Geometry: final body of the model. Coordinates: model frame, mm. A direction names the side the tool comes from. Give positions to 0.01 mm unless a question says otherwise; leave off trailing zeros. Write each loop counter-clockwise with the first axis right and the second up, starting at its lowest first coordinate (ties: lowest second). Pieces come first, ordered by that corner, then holes. Notation, with made-up numbers: (66, 81.25) -> (104, 81.25) arc R13 ccw to (104, 101.25) -> close; hole circle Ø4 at (47, -31.5). An arc over 180 degrees is marked (long way). Answer in a Markdown table with one row per item. Add a question column.
Item 1: Material intervals for probe 1 along X at (y, z) = (14, -23); probe 2 along Y at (x, z) = (-9.75, 12); probe 3 along Z at (x, y) = (-0.75, 15), sorted ascending. Write a range as from..to.
Item 2: Section query B-B on y = 20.25. Output: boundary loops of the cut face in (x, z), plus the area to 3 significant figures.
Item 3: Section query C-C on x = -1.75. Output: boundary loops of the cut face in (y, z).
Item 4: First-contact query: P1, Ø8, axis at x = -9, y = 6.5, coming from the -Z side; P2, Ø6, axis at x = -8, z = -9, coming from the +Y side; P3, Ø4, axis at y = 15, z = -12, coming from the +X side; P4, Ø3, axis at x = 11, y = 16.5, coming from the -Z side. Flat tips, straight axial feed; report the tip coordinate or a pass-through.
Item 5: Section query D-D on y = 15. Output: boundary loops of the cut face in (x, z).
Item 6: Draft query along Y for faces 1 (the flat face through (-0.133, 25.244, 25.986)), 2 (the flat face through (7.5, 16, 0)), 3 (the cylindrical face through (-11.2, 12.87, -14.32)), 4 (the flat face through (0, 0, 0)). Return one class per face: +Y half, -Y half, draft (parallel to the pull), parting line (faces both ways), or undercut.
Item 7: Section query A-A on z = 12.5. Output: boundary loops of the cut face in (x, y), plus the area to 3 significant figures.
Item 8: Access query for faces 5 (the flat face through (0, 21, -25)), 6 (the flat face through (-15, 16, 1)). Directions: +Z, -Z, +X, -X, +Y, -Y. A direction counts if a zero-diameter tool reaches every point of the face in a straight line with its end or side. Return the directions, or none.
```python
from build123d import *

# Parameters (mm, degrees)
SKETCH1_W           = 30
SKETCH1_H           = 80
BOSS_EXTRUDE1_DEPTH = 27
SKETCH5_W           = 30
SKETCH5_H           = 10
BOSS_EXTRUDE2_DEPTH = 6
SKETCH2_R           = 3.15
CUT_EXTRUDE1_DEPTH  = 40
FILLET5_R           = 40
FILLET6_R           = 40
FILLET7_R           = 2
FILLET8_R           = 2
SKETCH6_W           = 10
SKETCH6_H           = 6
CUT_EXTRUDE2_DEPTH  = 60.301649892
SKETCH7_W           = 15
SKETCH7_H           = 50
CUT_EXTRUDE3_DEPTH  = 19
FILLET9_R           = 10
CHAMFER1_SIZE       = 2
CHAMFER1_SIZE2      = 3.464101615


with BuildPart() as part:
    # Sketch1 → Boss-Extrude1 (new body)
    with BuildSketch(Plane(origin=(0, 0, 0), x_dir=(1, 0, 0), z_dir=(0, 1, 0))):
        Rectangle(SKETCH1_W, SKETCH1_H)
    extrude(amount=BOSS_EXTRUDE1_DEPTH)

    # Sketch5 → Boss-Extrude2 (add)
    with BuildSketch(Plane(origin=(0, 27, 0), x_dir=(1, 0, 0), z_dir=(0, 1, 0))):
        Rectangle(SKETCH5_W, SKETCH5_H)
    extrude(amount=BOSS_EXTRUDE2_DEPTH)

    # Sketch2 → Cut-Extrude1 (cut)
    with BuildSketch(Plane(origin=(15, 0, 0), x_dir=(0, 0, -1), z_dir=(1, 0, 0))):
        with Locations((-12, 15)):
            Circle(SKETCH2_R)
        with Locations(Location((12, 15, 0), (0, 0, 180))):
            Circle(SKETCH2_R)
    extrude(amount=-CUT_EXTRUDE1_DEPTH, mode=Mode.SUBTRACT)

    # Fillet5
    # the kernel refuses this fillet: 40 mm, written as the material it takes off along each edge
    with BuildSketch(Plane(origin=(109.571401597, 0, -40), x_dir=(0, 0, 1), z_dir=(-1, 0, 0))) as fillet5_piece_1:
        with BuildLine():
            CenterArc((37.828560639, 40), FILLET5_R, 198.965574989, 71.034425011)
            Line((0, 27), (-0.756571213, 26.74))
            ThreePointArc((-0.756571213, 26.74), (-0.8, 13.5), (-0.8, 0))
            Line((-0.8, 0), (0, -0.8))
            Line((0, -0.8), (37.828560639, -0.8))
            Line((37.828560639, -0.8), (37.828560639, 0))
        make_face()
    extrude(amount=219.142803194, mode=Mode.SUBTRACT)

    # Fillet6
    # the kernel refuses this fillet: 40 mm, written as the material it takes off along each edge
    with BuildSketch(Plane(origin=(-109.571401597, 0, 40), x_dir=(0, 1, 0), z_dir=(1, 0, 0))) as fillet6_piece_1:
        with BuildLine():
            CenterArc((40, -37.828560639), FILLET6_R, 108.965574989, 71.034425011)
            Line((0, -37.828560639), (-0.8, -37.828560639))
            Line((-0.8, -37.828560639), (-0.8, 0))
            Line((-0.8, 0), (0, 0.8))
            ThreePointArc((0, 0.8), (13.5, 0.8), (26.74, 0.756571213))
            Line((26.74, 0.756571213), (27, 0))
        make_face()
    extrude(amount=219.142803194, mode=Mode.SUBTRACT)

    # Fillet7
    fillet7_edges = [part.edges().sort_by_distance(p)[0] for p in [
        (0, 27, -40),
    ]]
    fillet(fillet7_edges, radius=FILLET7_R)

    # Fillet8
    fillet8_edges = [part.edges().sort_by_distance(p)[0] for p in [
        (0, 27, 40),
    ]]
    fillet(fillet8_edges, radius=FILLET8_R)

    # Sketch6 → Cut-Extrude2 (cut, through all)
    with BuildSketch(Plane(origin=(15, 0, 0), x_dir=(0, 0, -1), z_dir=(1, 0, 0))):
        with Locations((0, 30)):
            Rectangle(SKETCH6_W, SKETCH6_H)
    extrude(amount=-CUT_EXTRUDE2_DEPTH, mode=Mode.SUBTRACT)

    # Sketch7 → Cut-Extrude3 (cut)
    with BuildSketch(Plane(origin=(0, 27, 0), x_dir=(1, 0, 0), z_dir=(0, 1, 0))):
        Rectangle(SKETCH7_W, SKETCH7_H)
    extrude(amount=-CUT_EXTRUDE3_DEPTH, mode=Mode.SUBTRACT)

    # Fillet9
    fillet9_edges = [part.edges().sort_by_distance(p)[0] for p in [
        (0, 8, -25),
        (0, 8, 25),
    ]]
    fillet(fillet9_edges, radius=FILLET9_R)

    # Chamfer1
    chamfer1_edges = [part.edges().sort_by_distance(p)[0] for p in [
        (-7.5, 27, 0),
        (0, 27, 25),
        (7.5, 27, 0),
        (0, 27, -25),
    ]]
    chamfer1_side = [part.faces().sort_by_distance(p)[0] for p in [
        (-14.199914204, 27, 0),
    ]]
    chamfer(chamfer1_edges, length=CHAMFER1_SIZE, length2=CHAMFER1_SIZE2, reference=chamfer1_side[0])


solid = part.part
```
Findings below:
| question | item | result |
|---|---|---|
| 1 | probe 1 | x = -15..-7.5, 7.5..15 |
| 1 | probe 2 | y = 1.23..11.85, 18.15..27 |
| 1 | probe 3 | z = -33.4..-24.54, 24.54..33.4 |
| 2 | outline | (-15, -36.96) -> (15, -36.96) -> (15, 36.96) -> (-15, 36.96) -> close; hole (-7.5, -25) -> (7.5, -25) -> (7.5, 25) -> (-7.5, 25) -> close |
| 2 | area | 1,470 mm^2 |
| 3 | outline | (0, -2.17) arc R40 ccw to (24.21, -38.92) arc R2 ccw to (27, -37.09) -> (27, -27) -> (23.54, -25) -> (18, -25) arc R10 cw to (8, -15) -> (8, 15) arc R10 cw to (18, 25) -> (23.54, 25) -> (27, 27) -> (27, 37.09) arc R2 ccw to (24.21, 38.92) arc R40 ccw to (0, 2.17) -> close |
| 4 | P1 | stops at z = -29.19 |
| 4 | P2 | stops at y = 27 |
| 4 | P3 | passes through |
| 4 | P4 | stops at z = -35.58 |
| 5 | outline | (-15, -33.4) -> (15, -33.4) -> (15, -15.15) -> (7.5, -15.15) -> (7.5, -24.54) -> (-7.5, -24.54) -> (-7.5, -15.15) -> (-15, -15.15) -> close; (-15, -8.85) -> (-7.5, -8.85) -> (-7.5, 8.85) -> (-15, 8.85) -> close; (-15, 15.15) -> (-7.5, 15.15) -> (-7.5, 24.54) -> (7.5, 24.54) -> (7.5, 15.15) -> (15, 15.15) -> (15, 33.4) -> (-15, 33.4) -> close; (7.5, -8.85) -> (15, -8.85) -> (15, 8.85) -> (7.5, 8.85) -> close |
| 6 | face 1 | +Y half |
| 6 | face 2 | draft |
| 6 | face 3 | undercut |
| 6 | face 4 | -Y half |
| 7 | outline | (-15, 1.36) -> (15, 1.36) -> (15, 11.89) -> (7.5, 11.89) -> (7.5, 8) -> (-7.5, 8) -> (-7.5, 11.89) -> (-15, 11.89) -> close; (-15, 18.11) -> (-7.5, 18.11) -> (-7.5, 23.54) -> (-9.5, 27) -> (-15, 27) -> close; (7.5, 18.11) -> (15, 18.11) -> (15, 27) -> (9.5, 27) -> (7.5, 23.54) -> close |
| 7 | area | 384 mm^2 |
| 8 | face 5 | +Y |
| 8 | face 6 | +Z, -Z, -X, +Y, -Y |
